Source: CAD feature listing. Evaluate the final solid. Frame: model axes, mm. Give positions to 0.01 mm unless a question says otherwise; leave off trailing zeros. Order: outer loops, then holes, each group sorted by start corner. A loop starts at its lowest first (then second) coordinate and runs counter-clockwise, first axis right, second up. Notation, with made-up numbers: M 86.5,20 L 97.5,20 A16 cw 97.5,36 Z; hole C -30,75.25 d10. An arc over 180 degrees is marked long. Return JSON: item names as keys, results as strings.
from build123d import *

# Parameters (mm, degrees)
SKETCH2_W           = 24
SKETCH2_H           = 12
BOSS_EXTRUDE1_DEPTH = 4
SKETCH3_R           = 1.75
CUT_EXTRUDE1_DEPTH  = 5
FILLET1_R           = 1
CUT_EXTRUDE2_DEPTH  = 32


with BuildPart() as part:
    # Sketch2 → Boss-Extrude1 (new body)
    with BuildSketch(Plane.XY):
        with Locations((6.957345972, -2)):
            Rectangle(SKETCH2_W, SKETCH2_H)
    extrude(amount=BOSS_EXTRUDE1_DEPTH)

    # Sketch3 → Cut-Extrude1 (cut)
    with BuildSketch(Plane.XY.offset(4)):
        with Locations((6.957345972, -2)):
            Circle(SKETCH3_R)
    extrude(amount=-CUT_EXTRUDE1_DEPTH, mode=Mode.SUBTRACT)

    # Fillet1
    fillet1_edges = [part.edges().sort_by_distance(p)[0] for p in [
        (6.957345972, 4, 0),
        (6.957345972, -8, 0),
    ]]
    fillet(fillet1_edges, radius=FILLET1_R)

    # Sketch4 → Cut-Extrude2 (cut)
    with BuildSketch(Plane.ZY.offset(5.042654028)):
        with BuildLine():
            ThreePointArc((5.45, -4.9), (5.025304833, -3.874695167), (4, -3.45))
            Line((4, -3.45), (4, -6.35))
            ThreePointArc((4, -6.35), (5.025304833, -5.925304833), (5.45, -4.9))
        make_face()
        with BuildLine():
            Line((4, -6.35), (4, -3.45))
            ThreePointArc((4, -3.45), (2.55, -4.9), (4, -6.35))
        make_face()
        with BuildLine():
            ThreePointArc((4, -3.45), (5.025304833, -3.025304833), (5.45, -2))
            ThreePointArc((5.45, -2), (5.025304833, -0.974695167), (4, -0.55))
            Line((4, -0.55), (4, -3.45))
        make_face()
        with BuildLine():
            Line((4, -3.45), (4, -0.55))
            ThreePointArc((4, -0.55), (2.55, -2), (4, -3.45))
        make_face()
        with BuildLine():
            ThreePointArc((4, 2.35), (2.55, 0.9), (4, -0.55))
            Line((4, -0.55), (4, 2.35))
        make_face()
        with BuildLine():
            Line((4, 2.35), (4, -0.55))
            ThreePointArc((4, -0.55), (5.025304833, -0.125304833), (5.45, 0.9))
            ThreePointArc((5.45, 0.9), (5.025304833, 1.925304833), (4, 2.35))
        make_face()
    extrude(amount=-CUT_EXTRUDE2_DEPTH, mode=Mode.SUBTRACT)


solid = part.part
1. Section query D-D (z = 0.7). Return loops of the section in (x, y), then the cut area to 3 significant figures.
Evaluation:
{"outline": "M -5.04,-7.95 L 18.96,-7.95 L 18.96,3.95 L -5.04,3.95 Z; hole C 6.96,-2 d3.5", "area": "276 mm^2"}
2. First-contact query: pin 1 (5.5 mm diameter, centred on x = 6.96, y = -2, fed in from -Z). Flat tip, straight axial feed; report the tip coordinate or a pass-through.
Evaluation:
{"pin 1": "stops at z = 0"}
3. Ray query, probe 1 along X at (y, z) = (-2, 1.3); probe 2 along Y at (x, z) = (8.5, 2.7); probe 3 along X at (y, z) = (-0.5, 1.85). Return the intervals inside material, ascending.
Evaluation:
{"probe 1": "x = -5.04 to 5.21, 8.71 to 18.96", "probe 2": "y = -8 to -5.54, -4.26 to -2.83, -1.17 to 0.26, 1.54 to 4", "probe 3": "x = -5.04 to 6.06, 7.86 to 18.96"}
4. Section query B-B (z = 2.85). Return loops of the section in (x, y), then the cut area to 3 significant figures.
Evaluation:
{"outline": "M -5.04,-8 L 18.96,-8 L 18.96,-5.78 L -5.04,-5.78 Z; M -5.04,-4.02 L 18.96,-4.02 L 18.96,-2.88 L 8.47,-2.88 A1.75 cw 5.45,-2.88 L -5.04,-2.88 Z; M -5.04,-1.12 L 5.45,-1.12 A1.75 cw 8.47,-1.12 L 18.96,-1.12 L 18.96,0.02 L -5.04,0.02 Z; M -5.04,1.78 L 18.96,1.78 L 18.96,4 L -5.04,4 Z", "area": "157 mm^2"}
5. Section query A-A (y = -2). Return loops of the section in (x, z).
Evaluation:
{"outline": "M -5.04,0 L 5.21,0 L 5.21,2.55 L -5.04,2.55 Z; M 8.71,0 L 18.96,0 L 18.96,2.55 L 8.71,2.55 Z"}
6. Section query C-C (x = -3). Return loops of the section in (y, z).
Evaluation:
{"outline": "M -8,1 A1 ccw -7,0 L 3,0 A1 ccw 4,1 L 4,4 L 2.35,4 A1.45 cw -0.55,4 A1.45 cw -3.45,4 A1.45 cw -6.35,4 L -8,4 Z"}
7. Draft query along X for faces 1 (the face through (7, -7, 4)), 2 (the face through (8.627, -1.474, 1.584)), 3 (the face through (-5.043, -2, 2)). Return one class per face: pulls with the +X half, pulls with the -X half, needs draft (parallel to the pull), parting line crosses it, or undercut.
Evaluation:
{"face 1": "needs draft", "face 2": "undercut", "face 3": "pulls with the -X half"}
